```python
from build123d import *

# Parameters (mm, degrees)
SKETCH1_R                = 50
BOSS_EXTRUDE1_DEPTH      = 250
BOSS_EXTRUDE1_DEPTH_BACK = 100
BOSS_EXTRUDE2_DEPTH      = 55
SKETCH7_R                = 1.25
CUT_EXTRUDE4_DEPTH       = 75
CUT_EXTRUDE4_DEPTH_BACK  = 96
CUT_EXTRUDE5_DEPTH       = 96
CUT_EXTRUDE6_DEPTH       = 96
SKETCH10_R               = 1.25
CUT_EXTRUDE7_DEPTH       = 96


with BuildPart() as part:
    # Sketch1 → Boss-Extrude1 (new body, two sides)
    with BuildSketch(Plane.XY) as boss_extrude1_sk:
        Circle(SKETCH1_R)
        with BuildLine():
            Line((-44.955555556, 1.999506112), (-47.255555556, 1.999506112))
            Line((-47.255555556, 1.999506112), (-47.255555556, -1.999506112))
            Line((-47.255555556, -1.999506112), (-44.955555556, -1.999506112))
            ThreePointArc((-44.955555556, -1.999506112), (0, -45), (44.955555556, -1.999506112))
            Line((44.955555556, -1.999506112), (47.255555556, -1.999506112))
            Line((47.255555556, -1.999506112), (47.255555556, 1.999506112))
            Line((47.255555556, 1.999506112), (44.955555556, 1.999506112))
            ThreePointArc((44.955555556, 1.999506112), (0, 45), (-44.955555556, 1.999506112))
        make_face(mode=Mode.SUBTRACT)
    extrude(amount=BOSS_EXTRUDE1_DEPTH)
    extrude(boss_extrude1_sk.sketch, amount=-BOSS_EXTRUDE1_DEPTH_BACK)

    # Sketch3 → Boss-Extrude2 (add)
    with BuildSketch(Plane.XY.offset(250)):
        Polygon((28.2, 0), (28.2, 35.067934071), (35.640426485, 35.067934071), (35.640426485, -35.067934071), (28.2, -35.067934071), align=None)
    extrude(amount=BOSS_EXTRUDE2_DEPTH)

    # Sketch7 → Cut-Extrude4 (cut, two sides)
    with BuildSketch(Plane(origin=(35.640426485, 0, 0), x_dir=(0, 0, -1), z_dir=(1, 0, 0))) as cut_extrude4_sk:
        with Locations((-100, 0)):
            Circle(SKETCH7_R)
    extrude(amount=CUT_EXTRUDE4_DEPTH, mode=Mode.SUBTRACT)
    extrude(cut_extrude4_sk.sketch, amount=-CUT_EXTRUDE4_DEPTH_BACK, mode=Mode.SUBTRACT)

    # Sketch8 → Cut-Extrude5 (cut)
    with BuildSketch(Plane(origin=(35.640426485, 0, 0), x_dir=(0, 0, -1), z_dir=(1, 0, 0))):
        with BuildLine():
            Line((-287.5, 17.5), (-250, 35.067934071))
            Line((-250, 35.067934071), (-305, 35.067934071))
            Line((-305, 35.067934071), (-305, 0))
            ThreePointArc((-305, 0), (-299.874368671, 12.374368671), (-287.5, 17.5))
        make_face()
    extrude(amount=-CUT_EXTRUDE5_DEPTH, mode=Mode.SUBTRACT)

    # Sketch9 → Cut-Extrude6 (cut)
    with BuildSketch(Plane(origin=(35.640426485, 0, 0), x_dir=(0, 0, -1), z_dir=(1, 0, 0))):
        with BuildLine():
            Line((-287.5, -17.5), (-250, -35.067934071))
            Line((-250, -35.067934071), (-305, -35.067934071))
            Line((-305, -35.067934071), (-305, 0))
            ThreePointArc((-305, 0), (-299.874368671, -12.374368671), (-287.5, -17.5))
        make_face()
    extrude(amount=-CUT_EXTRUDE6_DEPTH, mode=Mode.SUBTRACT)

    # Sketch10 → Cut-Extrude7 (cut)
    with BuildSketch(Plane(origin=(35.640426485, 0, 0), x_dir=(0, 0, -1), z_dir=(1, 0, 0))):
        with Locations((-296.25, 0)):
            Circle(SKETCH10_R)
        with Locations((-287.5, 8.75)):
            Circle(SKETCH10_R)
        with Locations((-278.75, 0)):
            Circle(SKETCH10_R)
        with Locations((-287.5, -8.75)):
            Circle(SKETCH10_R)
    extrude(amount=-CUT_EXTRUDE7_DEPTH, mode=Mode.SUBTRACT)


solid = part.part
```
For this review, take the finished solid that the model builds, in its own axes (mm). A direction names the side the tool comes from. Coordinates: 2 decimals unless noted, no trailing zeros. Write each loop counter-clockwise with the first axis right and the second up, starting at its lowest first coordinate (ties: lowest second). Pieces come first, ordered by that corner, then holes.
(1) Add section D-D on x = -23.5. Give the boundary of the cut face in (y, z), then the cut area to 3 significant figures.
(2) Tool access review of faces 5 (the face through (-41, 19, -100)), 6 (the face through (45.4, 2.8, 250)), 7 (the face through (32, 0, 250)): name each direction out of +Z, -Z, +X, -X, +Y, -Y from which nothing blocks a thin tool from reaching the whole face with its end or side.
(3) Add section C-C on y = -21. Give the boundary of the cut face in (x, z), then the cut area to 3 significant figures.
(4) The part is to be moulded in two halves that separate along X. For faces 1 (the face through (31.97, -26.16, 269.01)), 2 (the face through (0.96, 44.99, 77.45)), 3 (the face through (28.2, 0, 271)), 4 (the face through (35.64, 0, 271)), say which applies: +X half, -X half, draft (parallel to the pull), parting line (faces both ways), or undercut.
(5) For pin 1 Ø2.5 at (x, z) = (-46.5, 38) entering from -Y; pin 2 Ø16.5 at (y, z) = (-11.5, 267) entering from +X; pin 3 Ø5 at (x, z) = (24, 69.5) entering from +Y, all flat-tipped, find the tip position at first contact; note any pin that passes through.
(6) Wall thickness on probe 1 along Y at (x, z) = (-0.5, 242); probe 2 along Z at (x, y) = (-47.95, 0); probe 3 along Z at (x, y) = (9, 46.5): over which ranges is each line inside the solid? List them lowest first.
(7) Add section A-A on x = 0. Give the boundary of the cut face in (y, z), then the cut area to 3 significant figures.
Answer sheet:
1. outline: (-44.13, -100) - (-38.38, -100) - (-38.38, 250) - (-44.13, 250) - close; (38.38, -100) - (44.13, -100) - (44.13, 250) - (38.38, 250) - close
1. area: 4,030 mm2
2. face 5: -Z, +X, -X, +Y, -Y
2. face 6: +Z, +X, +Y, -Y
2. face 7: -Z
3. outline: (-45.38, -100) - (-39.8, -100) - (-39.8, 250) - (-45.38, 250) - close; (28.2, 250) - (35.64, 250) - (35.64, 280.03) - (28.2, 280.03) - close; (39.8, -100) - (45.38, -100) - (45.38, 250) - (39.8, 250) - close
3. area: 4,130 mm2
4. face 1: draft
4. face 2: undercut
4. face 3: -X half
4. face 4: +X half
5. pin 1: stops at y = -21.27
5. pin 2: stops at x = 35.64
5. pin 3: stops at y = 45.14
6. probe 1: y = -50 to -45, 45 to 50
6. probe 2: z = -100 to 98.75, 101.25 to 250
6. probe 3: z = -100 to 250
7. outline: (-50, -100) - (-45, -100) - (-45, 250) - (-50, 250) - close; (45, -100) - (50, -100) - (50, 250) - (45, 250) - close
7. area: 3,500 mm2
